Part model, mm, in its own coordinate system. Face numbers are marked on the shaded views. A direction names the side the tool comes from. Coordinates: 2 decimals unless noted, no trailing zeros. Order: outer loops, then holes, each group sorted by start corner. A loop starts at its lowest first (then second) coordinate and runs counter-clockwise, first axis right, second up. Notation, with made-up numbers: M 8.25,-11 L 64.25,-11 A9 cw 64.25,-2 Z; hole C 12.25,5 d4. An arc over 180 degrees is marked long. Answer in a Markdown table with one row per item. Add a question column.
from build123d import *

# Parameters (mm, degrees)
SALIENTE_EXTRUIR1_DEPTH = 4
SALIENTE_EXTRUIR3_DEPTH = 13


with BuildPart() as part:
    # Croquis1 → Saliente-Extruir1 (new body)
    with BuildSketch(Plane(origin=(0, 0, 0), x_dir=(1, 0, 0), z_dir=(0, 1, 0))):
        with BuildLine():
            Line((-53.612307413, -2.177777778), (-41.166593192, -43.422222222))
            ThreePointArc((-41.166593192, -43.422222222), (0, -74), (41.166593192, -43.422222222))
            Line((41.166593192, -43.422222222), (53.612307413, -2.177777778))
            ThreePointArc((53.612307413, -2.177777778), (0, 70), (-53.612307413, -2.177777778))
        make_face()
    extrude(amount=SALIENTE_EXTRUIR1_DEPTH)

    # Croquis3 → Saliente-Extruir3 (add)
    with BuildSketch(Plane(origin=(0, 4, 0), x_dir=(1, 0, 0), z_dir=(0, 1, 0))):
        with BuildLine():
            Line((41.166593192, -43.422222222), (53.612307413, -2.177777778))
            ThreePointArc((53.612307413, -2.177777778), (0, 70), (-53.612307413, -2.177777778))
            Line((-53.612307413, -2.177777778), (-41.166593192, -43.422222222))
            ThreePointArc((-41.166593192, -43.422222222), (0, -74), (41.166593192, -43.422222222))
        make_face()
        with BuildLine():
            Line((38.294505295, -42.555555556), (50.740219516, -1.311111111))
            ThreePointArc((50.740219516, -1.311111111), (0, 67), (-50.740219516, -1.311111111))
            Line((-50.740219516, -1.311111111), (-38.294505295, -42.555555556))
            ThreePointArc((-38.294505295, -42.555555556), (0, -71), (38.294505295, -42.555555556))
        make_face(mode=Mode.SUBTRACT)
    extrude(amount=SALIENTE_EXTRUIR3_DEPTH)


solid = part.part
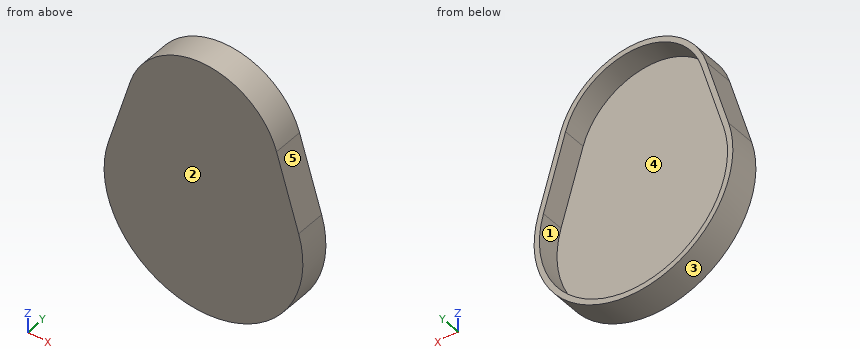
(1) Slice it at A-A (y = 9). List the corners of the cut face in (x, z).
(2) Slice it at C-C (z = -14). List the corners of the cut face in (x, y).
(3) Drop flat-ended pins along their axis: P1, Ø8, axis at x = 26.5, y = 8.5, coming from the -Z side; P2, Ø10, axis at x = 34, z = 8, coming from the +Y side; P3, Ø4, axis at y = 14.5, z = 38.5, coming from the +X side. Give the stop position or say it passes through.
(4) Slice it at D-D (y = 1.75). List the corners of the cut face in (x, z), and give its area (3 significant figures).
(5) Slice it at B-B (x = 0). List the corners of the cut face in (y, z), and give its area (3 significant figures).
(6) Wall check: line 1 (X direction, y = 11, z = -14); line 2 (Z direction, x = 0, y = 8.5); line 3 (Y direction, x = -5.5, z = -14.5). Give the ranges that are in metal, low to high.
(7) 3-axis set-ups, long thin cutter, end or side, ignore diameter. For the marked faces 1 and 2: which of +Z, -Z, +X, -X, +Y, -Y reach the whole face in a straight line?
(8) Pull direction Z, two halves, no side cores. Call the marked faces 3, 4 and 5: pulls with the +Z half, pulls with the -Z half, needs draft (parallel to the pull), parting line crosses it, or undercut.
Computed:
| question | item | result |
|---|---|---|
| 1 | outline | M -53.61,2.18 A56 ccw long 53.61,2.18 L 41.17,43.42 A43 ccw -41.17,43.42 Z; hole M -50.74,1.31 A53 ccw long 50.74,1.31 L 38.29,42.56 A40 ccw -38.29,42.56 Z |
| 2 | outline | M -56,0 L 56,0 L 56,17 L 53,17 L 53,4 L -53,4 L -53,17 L -56,17 Z |
| 3 | P1 | stops at z = -65.28 |
| 3 | P2 | stops at y = 4 |
| 3 | P3 | stops at x = 43.26 |
| 4 | outline | M -53.61,2.18 A56 ccw long 53.61,2.18 L 41.17,43.42 A43 ccw -41.17,43.42 Z |
| 4 | area | 12,500 mm^2 |
| 5 | outline | M 0,-70 L 17,-70 L 17,-67 L 4,-67 L 4,71 L 17,71 L 17,74 L 0,74 Z |
| 5 | area | 654 mm^2 |
| 6 | line 1 | x = -56 to -53, 53 to 56 |
| 6 | line 2 | z = -70 to -67, 71 to 74 |
| 6 | line 3 | y = 0 to 4 |
| 7 | face 1 | +Y |
| 7 | face 2 | +Z, -Z, +X, -X, -Y |
| 8 | face 3 | parting line crosses it |
| 8 | face 4 | undercut |
| 8 | face 5 | pulls with the +Z half |
